Read the model definition and answer for the solid it produces. Units are mm, in the model's axes. A direction names the side the tool comes from. Give positions to 0.01 mm unless a question says otherwise; leave off trailing zeros. Write each loop counter-clockwise with the first axis right and the second up, starting at its lowest first coordinate (ties: lowest second). Pieces come first, ordered by that corner, then holes. Notation, with made-up numbers: (7.5, 34) -> (35.5, 34) arc R20 cw to (35.5, 47) -> close; hole circle Ø1 at (-34.75, 14.5). An arc over 180 degrees is marked (long way). Put each result on its own line as item: value. Start each with the question number.
Solid Edge part; units mm, degrees
sketch "Sketch1" plane through (0, 0, 0) normal (0, -1, 0) x (1, 0, 0)
  line L0 (22, 14) -> (22, 0)
  line L1 (22, 0) -> (0, 0)
  line L2 (0, 0) -> (0, 21)
  line L3 (0, 21) -> (2.5, 21)
  line L4 (2.5, 21) -> (4.6838, 15)
  line L5 (4.6838, 15) -> (7.3162, 15)
  line L6 (7.3162, 15) -> (9.5, 21)
  line L7 (9.5, 21) -> (12, 21)
  line L8 (12, 21) -> (12, 14)
  line L9 (12, 14) -> (22, 14)
revolve "RevolvedProtrusion1" add sketch "Sketch1" angle 360 about axis through (22, 0, 0) along (-1, 0, 0)
sketch "Sketch2" plane through (0, 0, 0) normal (-1, 0, 0) x (0, 0, 1)
  line L0 (6.4, 1.5) -> (4.7697, 1.5)
  line L1 (6.4, 1.5) -> (6.4, -1.5)
  line L2 (6.4, -1.5) -> (4.7697, -1.5)
  arc A0 (4.7697, -1.5) -> (4.7697, 1.5) centre (0, 0) cw
extrude "Cutout1" cut sketch "Sketch2" along normal mid plane 276.6868
properties material "PVC"
1) For faces 5 (the face through (11, -1.5, 6)), 6 (the face through (0, -4, 4)), 7 (the face through (4.547, -15.01, -3.333)), determine the directions among +Z, -Z, +X, -X, +Y, -Y from which every point of the face is accessible in a straight line to the end or side of a thin tool.
2) A cutting plane is placed at D-D on x = 1.5. Give the vertices of the cut face in (y, z).
3) A cutting plane is placed at B-B on y = 0. Give the vertices of the cut face in (x, z), and give its area (3 significant figures).
4) A cutting plane is placed at C-C on x = 17.75. Give the vertices of the cut face in (y, z), and give its area (3 significant figures).
5) A cutting plane is placed at A-A on z = 0. Give the vertices of the cut face in (x, y), and give its area (3 significant figures).
6) Straight lines are drawn through the part: line 1 (Y direction, x = 4.75, z = 0); line 2 (Y direction, x = 14.25, z = 0); line 3 (Z direction, x = 15.5, y = 1). For each, find the intervals that lie inside material, in ascending order. Write a range as [from, to].
7) Each of these flat-tipped pins is pushed along its axis until it touches: pin 1 Ø4 at (x, z) = (10, 16.5) entering from -Y; pin 2 Ø5 at (x, z) = (4.5, -16) entering from +Y; pin 3 Ø1.3 at (x, z) = (6.5, 5.5) entering from +Y. Where does it stop, or does it pass through?
8) For a pull along X with two mould halves and no side action, classify faces 1 (the face through (17.07, 5.362, 12.932)), 2 (the face through (12, -14, 4)), 3 (the face through (6.018, -0.66, -14.985)), 4 (the face through (7.453, 9.356, -12.201)) as pulls with the +X half, pulls with the -X half, needs draft (parallel to the pull), parting line crosses it, or undercut.
Results found:
1. face 5: +X, -X
1. face 6: +Z, -Z, -X, +Y, -Y
1. face 7: none
2. outline: circle Ø42 at (0, 0); hole (-1.5, 4.77) arc R5 ccw (long way) to (1.5, 4.77) -> (1.5, 6.4) -> (-1.5, 6.4) -> close
3. outline: (0, -21) -> (2.5, -21) -> (4.68, -15) -> (7.32, -15) -> (9.5, -21) -> (12, -21) -> (12, -14) -> (22, -14) -> (22, -5) -> (0, -5) -> close; (0, 6.4) -> (22, 6.4) -> (22, 14) -> (12, 14) -> (12, 21) -> (9.5, 21) -> (7.32, 15) -> (4.68, 15) -> (2.5, 21) -> (0, 21) -> close
3. area: 475 mm²
4. outline: circle Ø28 at (0, 0); hole (-1.5, 4.77) arc R5 ccw (long way) to (1.5, 4.77) -> (1.5, 6.4) -> (-1.5, 6.4) -> close
4. area: 533 mm²
5. outline: (0, -21) -> (2.5, -21) -> (4.68, -15) -> (7.32, -15) -> (9.5, -21) -> (12, -21) -> (12, -14) -> (22, -14) -> (22, -5) -> (0, -5) -> close; (0, 5) -> (22, 5) -> (22, 14) -> (12, 14) -> (12, 21) -> (9.5, 21) -> (7.32, 15) -> (4.68, 15) -> (2.5, 21) -> (0, 21) -> close
5. area: 506 mm²
6. line 1: y = [-15, -5], [5, 15]
6. line 2: y = [-14, -5], [5, 14]
6. line 3: z = [-13.96, -4.9], [6.4, 13.96]
7. pin 1: stops at y = -15.19
7. pin 2: stops at y = 15.19
7. pin 3: stops at y = 14.19
8. face 1: needs draft
8. face 2: pulls with the +X half
8. face 3: undercut
8. face 4: undercut
